Geometry check sheet. Reference: drawing and pictorial views, mm from the part's lowest x, y, z. A direction names the side the tool comes from. Give positions to 0.01 mm unless a question says otherwise; leave off trailing zeros. Loops run counter-clockwise (first coordinate to the right, second up) from the corner with the lowest first, then second, coordinate; pieces in that order, holes last. Notation, with made-up numbers: M 43.5,33.25 L 64.5,33.25 A26 ccw 64.5,47.25 Z; hole C -31,11.5 d6. An arc over 180 degrees is marked long. Put each result on its own line as item: value. Start each with the question number.
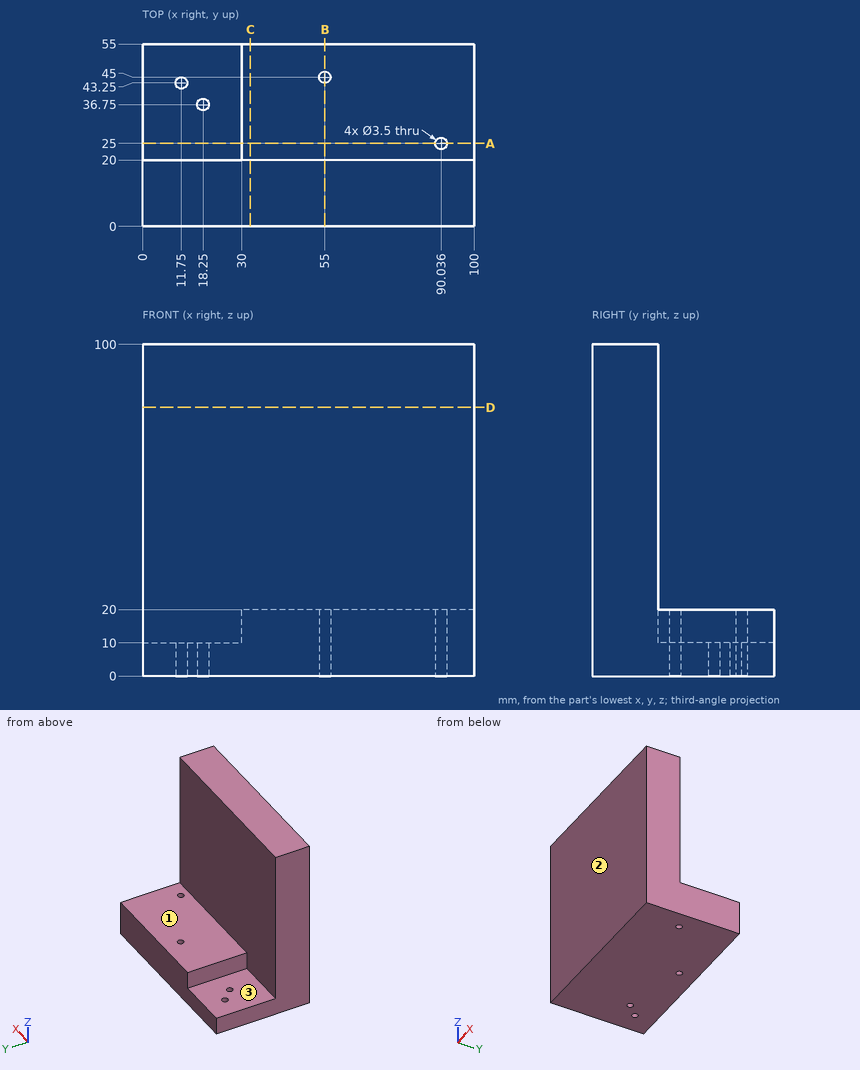
Q1. Section check C-C, the plane x = 32.5. Record the cut outline in (y, z), then the cut area to 3 significant figures.
Q2. Section check D-D, the plane z = 81. Record the cut outline in (x, y).
Q3. Section check B-B, the plane x = 55. Record the cut outline in (y, z), then the cut area to 3 significant figures.
Q4. Thickness scan on line 1 along Y through (x, z) = (18, 4); line 2 along X through (y, z) = (43, 8); line 3 along Y through (x, z) = (55, 14). Record the ranges inside material, lowest first. Write a range as [from, to].
Q5. Depth check by flat-ended pin: P1, Ø4.5, axis at x = 18.25, y = 36.75, coming from the +Z side; P2, Ø4.5, axis at x = 55, y = 45, coming from the +Z side. Enter the tip coordinate at first touch or a pass-through.
Q6. Section check A-A, the plane y = 25. Record the cut outline in (x, z).
Q7. Access from +Z, -Z, +X, -X, +Y, -Y to the whole of each face (thin tool, end or side, straight path). Record for the marked faces 1, 2 and 3.
Found:
1. outline: M 0,0 L 55,0 L 55,20 L 20,20 L 20,100 L 0,100 Z
1. area: 2,700 mm^2
2. outline: M 0,0 L 100,0 L 100,20 L 0,20 Z
3. outline: M 0,0 L 43.25,0 L 43.25,20 L 20,20 L 20,100 L 0,100 Z; M 46.75,0 L 55,0 L 55,20 L 46.75,20 Z
3. area: 2,630 mm^2
4. line 1: y = [0, 35.02], [38.48, 55]
4. line 2: x = [0, 10.02], [13.48, 100]
4. line 3: y = [0, 43.25], [46.75, 55]
5. P1: stops at z = 10
5. P2: stops at z = 20
6. outline: M 0,0 L 88.29,0 L 88.29,20 L 30,20 L 30,10 L 0,10 Z; M 91.79,0 L 100,0 L 100,20 L 91.79,20 Z
7. face 1: +Z, +X, -X, +Y
7. face 2: +Z, -Z, +X, -X, -Y
7. face 3: +Z, -X, +Y
